For this review, take the finished solid that the model builds, in its own axes (mm). A direction names the side the tool comes from. Coordinates: 2 decimals unless noted, no trailing zeros. Loops run counter-clockwise (first coordinate to the right, second up) from the corner with the lowest first, then second, coordinate; pieces in that order, holes last.
```python
from build123d import *

# Parameters (mm, degrees)
SKETCH1_W           = 25.4
SKETCH1_H           = 43.18
BOSS_EXTRUDE1_DEPTH = 6.35
SKETCH2_W           = 6.35
SKETCH2_H           = 12.7
BOSS_EXTRUDE2_DEPTH = 6.35
SKETCH3_W           = 12.7
SKETCH3_H           = 30.48
CUT_EXTRUDE1_DEPTH  = 30.484794386


with BuildPart() as part:
    # Sketch1 → Boss-Extrude1 (new body)
    with BuildSketch(Plane(origin=(0, 0, 0), x_dir=(1, 0, 0), z_dir=(0, 1, 0))):
        Rectangle(SKETCH1_W, SKETCH1_H)
    extrude(amount=BOSS_EXTRUDE1_DEPTH)

    # Sketch2 → Boss-Extrude2 (add)
    with BuildSketch(Plane.XZ):
        with Locations((-15.875, 12.7)):
            Rectangle(SKETCH2_W, SKETCH2_H)
        with Locations((15.875, 12.7)):
            Rectangle(SKETCH2_W, SKETCH2_H)
        with Locations((15.875, -12.7)):
            Rectangle(SKETCH2_W, SKETCH2_H)
        with Locations((-15.875, -12.7)):
            Rectangle(SKETCH2_W, SKETCH2_H)
    extrude(amount=-BOSS_EXTRUDE2_DEPTH)

    # Sketch3 → Cut-Extrude1 (cut, through all)
    with BuildSketch(Plane.XZ):
        Rectangle(SKETCH3_W, SKETCH3_H)
    extrude(amount=-CUT_EXTRUDE1_DEPTH, mode=Mode.SUBTRACT)


solid = part.part
```
Q1. For pin 1 Ø1.9 at (x, y) = (-17, 3) entering from -Z; pin 2 Ø1.9 at (y, z) = (1.5, 1) entering from +X; pin 3 Ø2 at (y, z) = (3, 20.5) entering from -X, all flat-tipped, find the tip position at first contact; note any pin that passes through.
Q2. Machinability: for faces 1 (the face through (-16, 3, -19.05)), 2 (the face through (-16, 3, 6.35)), 3 (the face through (6.35, 3, 0)), which of the approach directions +Z, -Z, +X, -X, +Y, -Y give a long, thin tool a straight path to every point of the face, cutting with its end or side? Answer none if there is none.
Q3. Consider section B-B (z = -9.5). State the section outline as (x, y) points.
Q4. Consider section C-C (y = 3.5). State the section outline as (x, z) points.
Q5. Consider section A-A (x = -5). State the section outline as (y, z) points, then the cut area to 3 significant figures.
Q6. Wall thickness on probe 1 along X at (y, z) = (5.5, 6.5); probe 2 along Z at (x, y) = (3.5, 0.75): over which ranges is each line inside the solid? List them lowest first.
Q7. The part is to be moulded in two halves that separate along X. For faces 4 (the face through (-6.35, 3, 0)), 5 (the face through (16, 3, -19.05)), 6 (the face through (-12.7, 3, 20)), say which applies: +X half, -X half, draft (parallel to the pull), parting line (faces both ways), or undercut.
Model answer:
1. pin 1: stops at z = -19.05
1. pin 2: stops at x = 12.7
1. pin 3: stops at x = -12.7
2. face 1: -Z, -X, +Y, -Y
2. face 2: -X, +Y, -Y
2. face 3: +Y, -Y
3. outline: (-19.05, 0) - (-6.35, 0) - (-6.35, 6.35) - (-19.05, 6.35) - close; (6.35, 0) - (19.05, 0) - (19.05, 6.35) - (6.35, 6.35) - close
4. outline: (-19.05, -19.05) - (-12.7, -19.05) - (-12.7, -21.59) - (12.7, -21.59) - (12.7, -19.05) - (19.05, -19.05) - (19.05, -6.35) - (12.7, -6.35) - (12.7, 6.35) - (19.05, 6.35) - (19.05, 19.05) - (12.7, 19.05) - (12.7, 21.59) - (-12.7, 21.59) - (-12.7, 19.05) - (-19.05, 19.05) - (-19.05, 6.35) - (-12.7, 6.35) - (-12.7, -6.35) - (-19.05, -6.35) - close; hole (-6.35, -15.24) - (6.35, -15.24) - (6.35, 15.24) - (-6.35, 15.24) - close
5. outline: (0, -21.59) - (6.35, -21.59) - (6.35, -15.24) - (0, -15.24) - close; (0, 15.24) - (6.35, 15.24) - (6.35, 21.59) - (0, 21.59) - close
5. area: 80.6 mm2
6. probe 1: x = -19.05 to -6.35, 6.35 to 19.05
6. probe 2: z = -21.59 to -15.24, 15.24 to 21.59
7. face 4: undercut
7. face 5: draft
7. face 6: -X half
